Check sheet for the drawn part. Datum: minimum x, y, z corner. Units: mm. A direction names the side the tool comes from. Round coordinates to 2 decimals unless told otherwise and drop trailing zeros. Write each loop counter-clockwise with the first axis right and the second up, starting at its lowest first coordinate (ties: lowest second). Pieces come first, ordered by that corner, then holes. Notation, with made-up numbers: M 14.5,26.5 L 30.5,26.5 A12 cw 30.5,37.5 Z; hole C 15,-16.75 d9. An arc over 180 degrees is marked long. One line per item, written item: value. Start each with the question number.
1. Scan lines: probe 1 along Z at (x, y) = (0.95, 1.75); probe 2 along Z at (x, y) = (2.6, 14.75) (3 decimals); probe 3 along Y at (x, z) = (1.25, 24.5). Record each from-to range of solid material in increasing order. Write a range as [from, to].
2. Section check C-C (z = 13.5). Record the boundary of the cut face in (x, y).
3. Section check A-A (x = 2.45). Record the boundary of the cut face in (y, z) (3 decimals).
4. Depth check by flat-ended pin: P1, Ø1.5, axis at x = 1, y = 7, coming from the +Z side (3 decimals); P2, Ø6, axis at y = 11.5, z = 13.5, coming from the -X side; P3, Ø0.8, axis at x = 1, y = 3.5, coming from the -Z side; P4, Ø1.5, axis at x = 0.5, y = 15.5, coming from the -Z side. Enter the tip coordinate at first touch or a pass-through.
5. Section check B-B (y = 16.5). Record the boundary of the cut face in (x, z) (1 decimal).
6. Access from +Z, -Z, +X, -X, +Y, -Y to the whole of each face (thin tool, end or side, straight path). Record for the marked faces 1, 2, 3, 4 and 5.
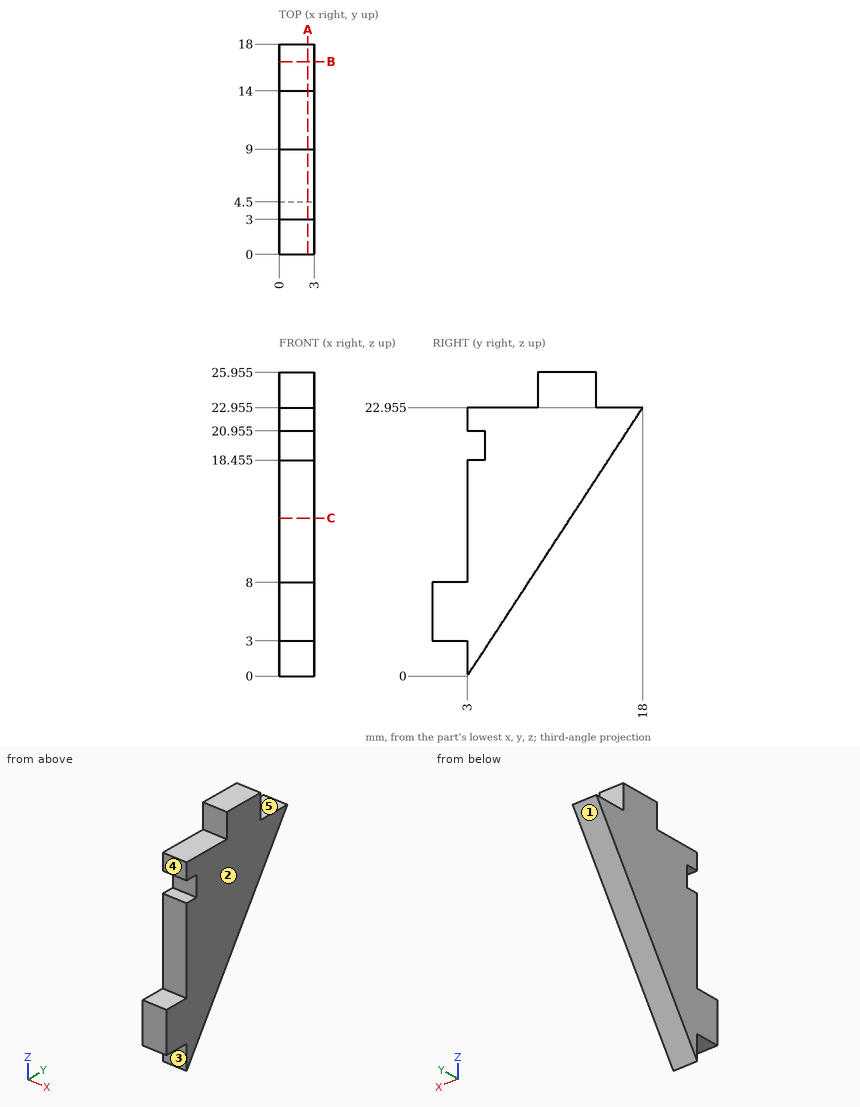
Result sheet:
1. probe 1: z = [3, 8]
1. probe 2: z = [17.981, 22.955]
1. probe 3: y = [9, 14]
2. outline: M 0,3 L 3,3 L 3,11.82 L 0,11.82 Z
3. outline: M 0,3 L 3,3 L 3,0 L 18,22.955 L 14,22.955 L 14,25.955 L 9,25.955 L 9,22.955 L 3,22.955 L 3,20.955 L 4.5,20.955 L 4.5,18.455 L 3,18.455 L 3,8 L 0,8 Z
4. P1: stops at z = 22.955
4. P2: stops at x = 0
4. P3: stops at z = 0.15
4. P4: stops at z = 17.98
5. outline: M 0,20.7 L 3,20.7 L 3,23 L 0,23 Z
6. face 1: -Z, +X, -X, +Y
6. face 2: +Z, -Z, +X, +Y, -Y
6. face 3: -Z, +X, -X, -Y
6. face 4: +Z, +X, -X, -Y
6. face 5: +Z, +X, -X, +Y
